from build123d import *

# Parameters (mm, degrees)
BOSS_EXTRUDE1_DEPTH = 50
SKETCH2_R           = 7.5
BOSS_EXTRUDE2_DEPTH = 10
FILLET1_R           = 10
CHAMFER1_SIZE       = 2


with BuildPart() as part:
    # Sketch1 → Boss-Extrude1 (new body, symmetric)
    with BuildSketch(Plane(origin=(0, 0, 0), x_dir=(1, 0, 0), z_dir=(0, 1, 0))):
        with BuildLine():
            Line((-56.319582284, 105.962751245), (0, 0))
            Line((0, 0), (57.1, 0))
            Line((57.1, 0), (78.545069205, 10))
            Line((78.545069205, 10), (69.74571647, 28.870272836))
            ThreePointArc((69.74571647, 28.870272836), (58.104205428, 39.537752317), (42.329366947, 38.849007995))
            Line((42.329366947, 38.849007995), (12.63007346, 25))
            Line((12.63007346, 25), (-22.414079104, 100.152427697))
            ThreePointArc((-22.414079104, 100.152427697), (-34.192619771, 110.666026263), (-49.926831892, 109.360521003))
            Line((-49.926831892, 109.360521003), (-56.319582284, 105.962751245))
        make_face()
    extrude(amount=BOSS_EXTRUDE1_DEPTH, both=True)

    # Sketch2 → Boss-Extrude2 (add)
    with BuildSketch(Plane.XY):
        with Locations((28.55, 0)):
            Circle(SKETCH2_R)
    extrude(amount=BOSS_EXTRUDE2_DEPTH)

    # Fillet1
    fillet1_edges = [part.edges().sort_by_distance(p)[0] for p in [
        (74.145392838, -50, -19.435136418),
        (-53.123207088, -50, -107.661636124),
        (74.145392838, 50, -19.435136418),
        (58.104205428, 50, -39.537752317),
        (27.479720204, 50, -31.924503997),
        (-4.892002822, 50, -62.576213849),
        (-34.192619771, 50, -110.666026263),
        (-53.123207088, 50, -107.661636124),
        (-34.192619771, -50, -110.666026263),
        (-4.892002822, -50, -62.576213849),
        (27.479720204, -50, -31.924503997),
        (58.104205428, -50, -39.537752317),
    ]]
    fillet(fillet1_edges, radius=FILLET1_R)

    # Chamfer1
    chamfer1_edges = [part.edges().sort_by_distance(p)[0] for p in [
        (-56.319582284, 0, -105.962751245),
        (-25.81314188, -50, -48.566260987),
        (-25.81314188, 50, -48.566260987),
        (-54.944946973, 47.071067812, -103.376436971),
        (-54.944946973, -47.071067812, -103.376436971),
    ]]
    chamfer(chamfer1_edges, length=CHAMFER1_SIZE)


solid = part.part
Can you work these out from the model? Positions are in its coordinate system, mm. A direction names the side the tool comes from. Give positions to 0.01 mm unless a question says otherwise; leave off trailing zeros. Order: outer loops, then holes, each group sorted by start corner. A loop starts at its lowest first (then second) coordinate and runs counter-clockwise, first axis right, second up. Notation, with made-up numbers: M 0.25,57 L 47.25,57 A17 ccw 47.25,80 Z; hole C -13.75,77.5 d1. An arc over 180 degrees is marked long. Use one line per item in the form item = value. Start each with the question number.
Item 1: For faces 5 (the flat face through (27.688, 0.56, -32.021)), 6 (the flat face through (74.21, 0.56, -19.3)), which set-ups out of +Z, -Z, +X, -X, +Y, -Y let a thin tool reach every point of the face, with its end or its side?
Item 2: If we section it at B-B (z = -3.5): Write out the boundary of the cut face in (x, y).
Item 3: Will these pins go through, and if not, where does the flat tip stop? pin 1 Ø12 at (x, y) = (32.5, -19.5) entering from +Z; pin 2 Ø10 at (y, z) = (21.5, -98.5) entering from -X; pin 3 Ø12 at (y, z) = (-26, -12.5) entering from -X.
Item 4: If I drill on line 1 along X through (y, z) = (-11, -36.5); line 2 along X through (y, z) = (-40, -33); line 3 along X through (y, z) = (-6, -59), over which ranges is the centre line in solid material (lowest first)?
Item 5: We'd pull the mould along X, two halves only. Please class faces 1 (the cylindrical face through (28.255, 47.148, -28.968)), 2 (the cylindrical face through (35.48, -2.87, 4.93)), 3 (the cylindrical face through (-5.78, 47.15, -57.36)), 4 (the flat face through (28, 12, 0)): +X half, -X half, draft (parallel to the pull), parting line (faces both ways), or undercut.
Item 6: If we section it at C-C (y = 0): Write out the boundary of the cut face in (x, z), then the cut area to 3 significant figures.
Item 7: If we section it at A-A (y = -13): Write out the boundary of the cut face in (x, z), then the cut area to 3 significant figures.
Outcome:
q1.face_5 = -Z, +Y, -Y
q1.face_6 = -Z, +X, +Y, -Y
q2.outline = M -1.86,-48 L 0.4,-50 L 64.61,-50 L 64.61,50 L 0.4,50 L -1.86,48 Z
q3.pin_1 = 0
q3.pin_2 = -55.01
q3.pin_3 = -9.83
q4.line_1 = -19.4 to 7.27, 37.29 to 63.63
q4.line_2 = -17.54 to 8.9, 29.79 to 67.19
q4.line_3 = -31.36 to -3.22
q5.face_1 = undercut
q5.face_2 = parting line
q5.face_3 = undercut
q5.face_4 = draft
q6.outline = M -55.38,-104.2 L -54.55,-106.9 L -49.93,-109.36 A20 ccw -22.41,-100.15 L 12.63,-25 L 42.33,-38.85 A20.63 ccw 69.75,-28.87 L 78.55,-10 L 57.1,0 L 36.05,0 L 36.05,10 L 21.05,10 L 21.05,0 L 0,0 Z
q6.area = 5,110 mm2
q7.outline = M -55.38,-104.2 L -54.55,-106.9 L -49.93,-109.36 A20 ccw -22.41,-100.15 L 12.63,-25 L 42.33,-38.85 A20.63 ccw 69.75,-28.87 L 78.55,-10 L 57.1,0 L 0,0 Z
q7.area = 4,960 mm2
